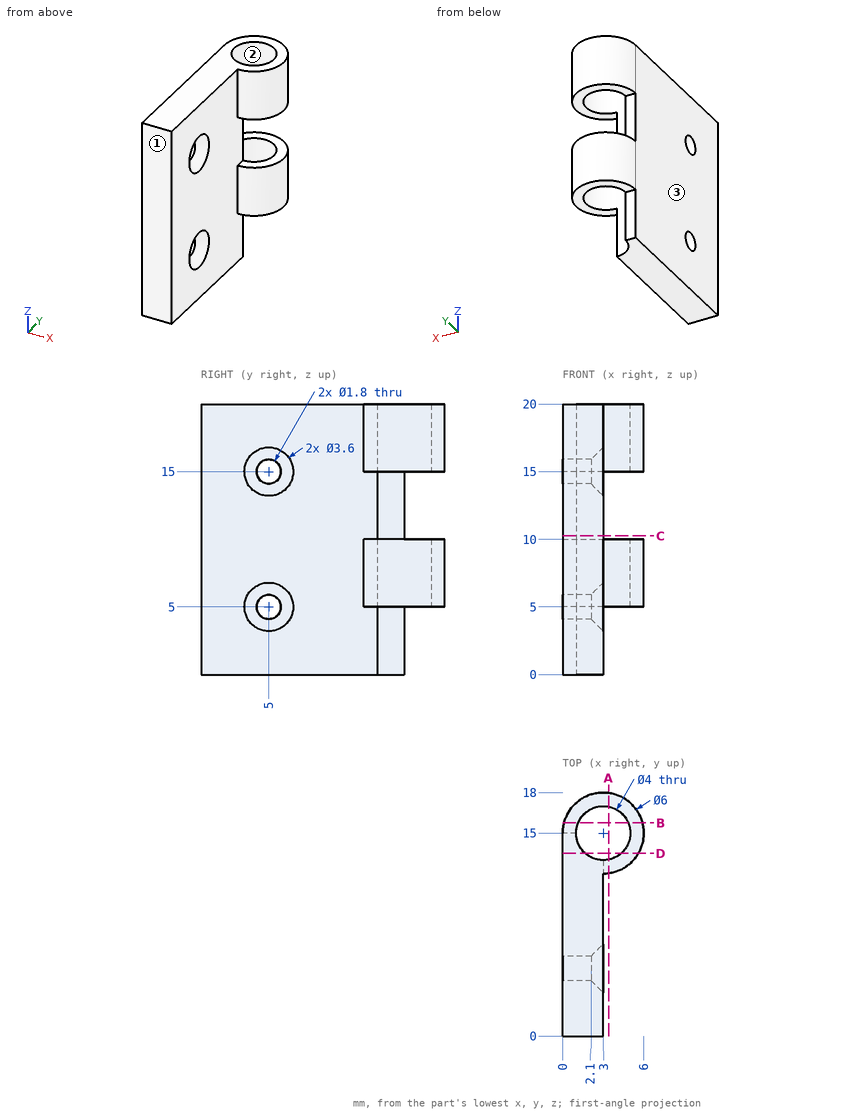
Geometry: see drawing. Coordinates: mm, zero at the bounding-box minimum. Coordinates: 2 decimals unless noted, no trailing zeros. Loops run counter-clockwise (first coordinate to the right, second up) from the corner with the lowest first, then second, coordinate; pieces in that order, holes last. Notation, with made-up numbers: (-39.5, -13) -> (-3.5, -13) arc R26 cw to (-3.5, 4) -> close; hole circle Ø6 at (-19.5, 21.25). An arc over 180 degrees is marked (long way). Write item = value, one per line. Start each with the question number.
Item 1: Cut plane C-C, the plane z = 10.25. Return loops of the section in (x, y).
Item 2: Cut plane A-A, the plane x = 3.4. Return loops of the section in (y, z).
Item 3: First-contact query: P1, Ø0.8, axis at x = 0.5, z = 13.5, coming from the +Y side; P2, Ø1.1, axis at y = 5, z = 5, coming from the -X side; P3, Ø10.5, axis at y = 9, z = 12, coming from the +X side. Flat tips, straight axial feed; report the tip coordinate or a pass-through.
Item 4: Cut plane D-D, the plane y = 13.5. Return loops of the section in (x, z).
Item 5: Mould query, pull axis Y, two halves, no side actions, for the marked faces 1, 2 and 3. Classes: pulls with the +Y half, pulls with the -Y half, needs draft (parallel to the pull), parting line crosses it, or undercut.
Item 6: Cut plane B-B, the plane y = 15.75. Return loops of the section in (x, z).
Item 7: Material intervals for line 1 (Z direction, x = 1.9, y = 17); line 2 (Z direction, x = 1.2, y = 5); line 3 (X direction, y = 15, z = 7.5), sorted ascending.
Ans:
q1.outline = (0, 0) -> (3, 0) -> (3, 13) arc R2 cw to (1, 15) -> (0, 15) -> close
q2.outline = (12.03, 5) -> (13.04, 5) -> (13.04, 10) -> (12.03, 10) -> close; (12.03, 15) -> (13.04, 15) -> (13.04, 20) -> (12.03, 20) -> close; (16.96, 5) -> (17.97, 5) -> (17.97, 10) -> (16.96, 10) -> close; (16.96, 15) -> (17.97, 15) -> (17.97, 20) -> (16.96, 20) -> close
q3.P1 = 15
q3.P2 = through
q3.P3 = 5.77
q4.outline = (0, 0) -> (1.68, 0) -> (1.68, 20) -> (0, 20) -> close; (4.32, 5) -> (5.6, 5) -> (5.6, 10) -> (4.32, 10) -> close; (4.32, 15) -> (5.6, 15) -> (5.6, 20) -> (4.32, 20) -> close
q5.face_1 = pulls with the -Y half
q5.face_2 = undercut
q5.face_3 = needs draft
q6.outline = (0.1, 5) -> (1.15, 5) -> (1.15, 10) -> (0.1, 10) -> close; (0.1, 15) -> (1.15, 15) -> (1.15, 20) -> (0.1, 20) -> close; (4.85, 5) -> (5.9, 5) -> (5.9, 10) -> (4.85, 10) -> close; (4.85, 15) -> (5.9, 15) -> (5.9, 20) -> (4.85, 20) -> close
q7.line_1 = 5 to 10, 15 to 20
q7.line_2 = 0 to 4.1, 5.9 to 14.1, 15.9 to 20
q7.line_3 = 0 to 1, 5 to 6
